```python
from build123d import *

# Parameters (mm, degrees)
SKETCH1_W           = 200
SKETCH1_H           = 108
BOSS_EXTRUDE1_DEPTH = 1
SKETCH3_W           = 16
SKETCH3_H           = 27
BOSS_EXTRUDE2_DEPTH = 1
CUT_EXTRUDE1_REACH  = 209.858
SKETCH4_R           = 3
FILLET2_R           = 4
CUT_EXTRUDE2_REACH  = 209.858
SKETCH6_R           = 1.65
FILLET3_R           = 4
SKETCH7_W           = 1
SKETCH7_H           = 31
BOSS_EXTRUDE3_DEPTH = 15


with BuildPart() as part:
    # Sketch1 → Boss-Extrude1 (new body)
    with BuildSketch(Plane.YZ):
        Rectangle(SKETCH1_W, SKETCH1_H)
    extrude(amount=-BOSS_EXTRUDE1_DEPTH)

    # Sketch3 → Boss-Extrude2 (add)
    with BuildSketch(Plane(origin=(0, 100, 0), x_dir=(-1, 0, 0), z_dir=(0, 1, 0))):
        with Locations((9, 40.5)):
            Rectangle(SKETCH3_W, SKETCH3_H)
    boss_extrude2 = extrude(amount=-BOSS_EXTRUDE2_DEPTH)

    # Sketch4 → Cut-Extrude1 (cut, up to next)
    with BuildSketch(Plane(origin=(0, 100, 0), x_dir=(-1, 0, 0), z_dir=(0, 1, 0)), mode=Mode.PRIVATE) as cut_extrude1_sk1:
        with Locations(Location((11, 47.5, 0), (0, 0, 90))):
            Circle(SKETCH4_R)
    cut_extrude1_tool1 = extrude(cut_extrude1_sk1.sketch, amount=-CUT_EXTRUDE1_REACH, mode=Mode.PRIVATE) & part.part
    add(cut_extrude1_tool1.solids().sort_by_distance((-11, 100, 47.5))[0], mode=Mode.SUBTRACT)

    # Fillet2
    fillet2_edges = [part.edges().sort_by_distance(p)[0] for p in [
        (-17, 99.5, 54),
        (-17, 99.5, 27),
    ]]
    fillet(fillet2_edges, radius=FILLET2_R)

    # Mirror1: Boss-Extrude2 across plane
    add(boss_extrude2.mirror(Plane.ZX))

    # Sketch6 → Cut-Extrude2 (cut, up to next)
    with BuildSketch(Plane.XZ.offset(100), mode=Mode.PRIVATE) as cut_extrude2_sk1:
        with Locations(Location((-11, 47.5, 0), (0, 0, 270))):
            Circle(SKETCH6_R)
    cut_extrude2_tool1 = extrude(cut_extrude2_sk1.sketch, amount=-CUT_EXTRUDE2_REACH, mode=Mode.PRIVATE) & part.part
    add(cut_extrude2_tool1.solids().sort_by_distance((-11, -100, 47.5))[0], mode=Mode.SUBTRACT)

    # Fillet3
    fillet3_edges = [part.edges().sort_by_distance(p)[0] for p in [
        (-17, -99.5, 27),
        (-17, -99.5, 54),
    ]]
    fillet(fillet3_edges, radius=FILLET3_R)

    # Sketch7 → Boss-Extrude3 (add, symmetric)
    with BuildSketch(Plane.XY.offset(54)):
        with Locations((-0.5, 0)):
            Rectangle(SKETCH7_W, SKETCH7_H)
    extrude(amount=BOSS_EXTRUDE3_DEPTH, both=True)


solid = part.part
```
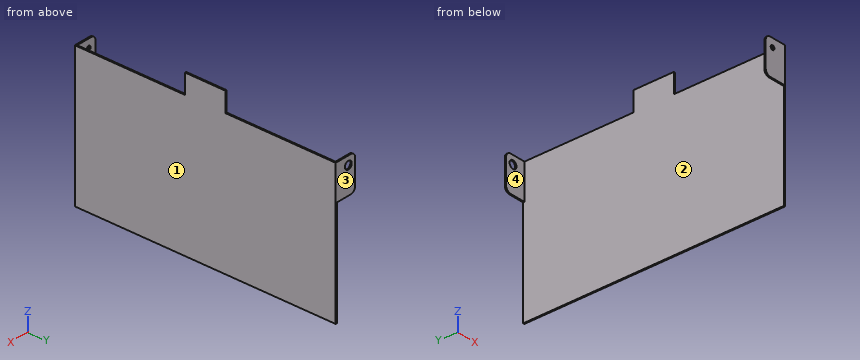
The model under review builds one solid part; all positions refer to its coordinate system, in mm. Face numbers are marked on the shaded views. Round coordinates to 2 decimals unless told otherwise and drop trailing zeros. Order: outer loops, then holes, each group sorted by start corner. A loop starts at its lowest first (then second) coordinate and runs counter-clockwise, first axis right, second up.
(1) Take a section at A-A, the plane x = -4.5. State the section outline as (y, z) points, plus the area to 3 significant figures.
Working result:
outline: (-100, 27) - (-99, 27) - (-99, 54) - (-100, 54) - close; (99, 27) - (100, 27) - (100, 54) - (99, 54) - close
area: 54.0 mm2
(2) Wall thickness on L1, parallel to Y at x = -7.5, z = 37.5; L2, parallel to X at y = -99.55, z = 47.5; L3, parallel to X at y = 99.8, z = 47.5: over which ranges is each line inside the solid? List them lowest first.
Working result:
L1: y = -100 to -99, 99 to 100
L2: x = -17 to -12.65, -9.35 to 0
L3: x = -17 to -14, -8 to 0
(3) Take a section at B-B, the plane y = -21. State the section outline as (x, z) points.
Working result:
outline: (-1, -54) - (0, -54) - (0, 54) - (-1, 54) - close
(4) Mouldability with a two-part tool opening along Y and no side actions: class the marked faces 1, 2, 3 and 4 as released by +Y, released by -Y, zero draft, split by the parting line, or undercut.
Working result:
face 1: zero draft
face 2: undercut
face 3: released by +Y
face 4: undercut
(5) For P1, Ø4, axis at x = -11, z = 47.5, coming from the +Y side; P2, Ø5, axis at y = 80, z = -16.5, coming from the -X side; P3, Ø0.5, axis at x = -9.5, y = 99.5, coming from the -Z side, all flat-tipped, find the tip position at first contact; note any pin that passes through.
Working result:
P1: stops at y = -99
P2: stops at x = -1
P3: stops at z = 27
(6) Take a section at C-C, the plane z = -46. State the section outline as (x, y) points, plus the area to 3 significant figures.
Working result:
outline: (-1, -100) - (0, -100) - (0, 100) - (-1, 100) - close
area: 200 mm2
